```python
from build123d import *

# Parameters (mm, degrees)
F0_W     = 6
F0_H     = 64
F1_DEPTH = 3
F2_R     = 1.5
F3_DEPTH = 5
F4_R     = 1.5
F5_DEPTH = 24.5


with BuildPart() as f1:
    # F0 (on Front) → F1 (new body)
    with BuildSketch(Plane.XZ):
        Rectangle(F0_W, F0_H)
    extrude(amount=F1_DEPTH)

    # F2 (on face) → F3 (cut)
    with BuildSketch(Plane.XZ.offset(3)):
        with Locations((0, 2)):
            Circle(F2_R)
        with Locations((0, 22)):
            Circle(F2_R)
    extrude(amount=-F3_DEPTH, mode=Mode.SUBTRACT)

    # F4 (on face) → F5 (join)
    with BuildSketch(Plane.XZ.offset(3)):
        with Locations((0, -28)):
            Circle(F4_R)
    extrude(amount=-F5_DEPTH)


solid = f1.part
```
Could you check a few things on this model? Use its own coordinates, in mm. A direction names the side the tool comes from. Give positions to 0.01 mm unless a question says otherwise; leave off trailing zeros. Loops run counter-clockwise (first coordinate to the right, second up) from the corner with the lowest first, then second, coordinate; pieces in that order, holes last. Notation, with made-up numbers: (20.25, 19) - (30.25, 19) arc R35 ccw to (30.25, 56) - close; hole circle Ø10 at (35.25, 7.25). An arc over 180 degrees is marked (long way). Answer in a Markdown table with one row per item. Add a question column.
Q1. For pin 1 (2 mm diameter, centred on x = 2, y = 14, fed in from +Z); pin 2 (2 mm diameter, centred on x = -0.5, y = 12.5, fed in from +Z); pin 3 (1.5 mm diameter, centred on x = 1, y = 7.5, fed in from -Z), each with a flat end and sliding along its axis, tell me the tip position at first contact or that it passes through.
Q2. If we section it at C-C (z = -28): List the corners of the cut face in (x, y) for me.
Q3. If we section it at D-D (y = 7.5): List the corners of the cut face in (x, z) for me, plus the area to 3 significant figures.
Q4. If we section it at A-A (z = 22): List the corners of the cut face in (x, y) for me.
Q5. Which directions (+Z, -Z, +X, -X, +Y, -Y) give clear straight access to the entire face, cutting with the end or side of a thin tool? Please do faces 1 (the face through (-0.195, 10.599, -26.513)), 2 (the face through (0, -1, 32)).
Q6. Please list where these lines run through material, in increasing order: L1, parallel to Z at x = 0, y = -1.9; L2, parallel to Y at x = 1.7, z = -12; L3, parallel to Z at x = 0.7, y = 14.5. Write a range as from..to.
Q7. If we section it at B-B (x = 0): List the corners of the cut face in (y, z) for me, plus the area to 4 significant figures.
Q8. We'd pull the mould along Z, two halves only. Please class faces 3 (the face through (-0.325, -1.521, 0.536)), 4 (the face through (0, -1, -32)), 5 (the face through (-3, -1, 0)), 6 (the face through (-0.195, -1.521, 23.487)): +Z half, -Z half, draft (parallel to the pull), parting line (faces both ways), or undercut.
The answers:
| question | item | result |
|---|---|---|
| 1 | pin 1 | stops at z = -26.88 |
| 1 | pin 2 | stops at z = -26.5 |
| 1 | pin 3 | stops at z = -29.48 |
| 2 | outline | (-3, -3) - (3, -3) - (3, 0) - (1.5, 0) - (1.5, 21.5) - (-1.5, 21.5) - (-1.5, 0) - (-3, 0) - close |
| 3 | outline | circle Ø3 at (0, -28) |
| 3 | area | 7.07 mm^2 |
| 4 | outline | (-3, -3) - (-1.5, -3) - (-1.5, 0) - (-3, 0) - close; (1.5, -3) - (3, -3) - (3, 0) - (1.5, 0) - close |
| 5 | face 1 | +Y |
| 5 | face 2 | +Z, +X, -X, +Y, -Y |
| 6 | L1 | z = -32..0.5, 3.5..20.5, 23.5..32 |
| 6 | L2 | y = -3..0 |
| 6 | L3 | z = -29.33..-26.67 |
| 7 | outline | (-3, -32) - (0, -32) - (0, -29.5) - (21.5, -29.5) - (21.5, -26.5) - (0, -26.5) - (0, 0.5) - (-3, 0.5) - close; (-3, 3.5) - (0, 3.5) - (0, 20.5) - (-3, 20.5) - close; (-3, 23.5) - (0, 23.5) - (0, 32) - (-3, 32) - close |
| 7 | area | 238.5 mm^2 |
| 8 | face 3 | undercut |
| 8 | face 4 | -Z half |
| 8 | face 5 | draft |
| 8 | face 6 | undercut |
